Autodesk Inventor part; units mm, degrees
ref_plane "YZ Plane" through (0, 0, 0) normal (1, 0, 0) x (0, 1, 0)
ref_plane "XZ Plane" through (0, 0, 0) normal (0, 1, 0) x (-1, 0, 0)
ref_plane "XY Plane" through (0, 0, 0) normal (0, 0, 1) x (1, 0, 0)
sketch "Sketch1" plane through (0, 0, 0) normal (0, 0, 1) x (1, 0, 0)
  line L0 (-4.55, 7.5) -> (4.55, 7.5)
  line L1 (4.55, 7.5) -> (4.55, -7.5)
  line L2 (4.55, -7.5) -> (-4.55, -7.5)
  line L3 (-4.55, -7.5) -> (-4.55, 7.5)
  line L4 (-4.55, 7.5) -> (4.55, -7.5) construction
  line L5 (4.55, 7.5) -> (-4.55, -7.5) construction
  line L6 (-2.05, -2.05) -> (2.05, -2.05)
  line L7 (2.05, -2.05) -> (2.05, 2.05)
  line L8 (2.05, 2.05) -> (-2.05, 2.05)
  line L9 (-2.05, 2.05) -> (-2.05, -2.05)
  line L10 (-2.05, -2.05) -> (2.05, 2.05) construction
  line L11 (2.05, -2.05) -> (-2.05, 2.05) construction
  line L12 (-4.55, 7.5) -> (-16.55, 7.5)
  line L13 (-16.55, 7.5) -> (-16.55, 6)
  line L14 (-16.55, 6) -> (-4.55, 6)
  line L15 (-4.55, 6) -> (-4.55, 7.5)
  line L16 (-4.55, -7.5) -> (-16.55, -7.5)
  line L17 (-16.55, -7.5) -> (-16.55, -6)
  line L18 (-16.55, -6) -> (-4.55, -6)
  line L19 (-4.55, -6) -> (-4.55, -7.5)
  line L20 (4.55, 7.5) -> (16.55, 7.5)
  line L21 (16.55, 7.5) -> (16.55, 6)
  line L22 (16.55, 6) -> (4.55, 6)
  line L23 (4.55, 6) -> (4.55, 7.5)
  line L24 (4.55, -7.5) -> (16.55, -7.5)
  line L25 (16.55, -7.5) -> (16.55, -6)
  line L26 (16.55, -6) -> (4.55, -6)
  line L27 (4.55, -6) -> (4.55, -7.5)
  point P0 (0, 0)
  point P1 (-4.55, 6)
  point P2 (-4.55, -6)
  point P3 (4.55, 6)
  dimension "d0" = 15
  dimension "d1" = 9.1
  dimension "d2" = 4.1
  dimension "d3" = 4.1
  dimension "d4" = 12
  dimension "d5" = 1.5
  dimension "d8" = 1.5
  dimension "d9" = 12
  dimension "d10" = 12
  dimension "d11" = 1.5
  dimension "d12" = 12
extrude "Extrusion1" add sketch "Sketch1" along normal blind 10
sketch "Sketch2" plane through (0, 0, 10) normal (0, 0, 1) x (1, 0, 0)
  point P0 (0, 0)
fillet "Fillet1" radius 2 8 edges at (-16.55, 6.75, 10) (-16.55, -6.75, 10) (16.55, -6.75, 10) (16.55, 6.75, 10) (16.55, 6.75, 0) (-16.55, 6.75, 0) (-16.55, -6.75, 0) (16.55, -6.75, 0)
sketch "Sketch3" plane through (0, 0, 0) normal (0, 0, -1) x (-1, 0, 0)
  line L0 (-2.05, 5.05) -> (2.05, 5.05)
  line L1 (2.05, 5.05) -> (2.05, 3.55)
  line L2 (2.05, 3.55) -> (-2.05, 3.55)
  line L3 (-2.05, 3.55) -> (-2.05, 5.05)
  line L4 (-2.05, -3.55) -> (2.05, -3.55)
  line L5 (2.05, -3.55) -> (2.05, -5.05)
  line L6 (2.05, -5.05) -> (-2.05, -5.05)
  line L7 (-2.05, -5.05) -> (-2.05, -3.55)
  line L8 (-2.05, 2.05) -> (-2.05, -2.05)
  line L9 (2.05, -2.05) -> (2.05, 2.05)
  line L10 (2.05, 2.05) -> (-2.05, 2.05)
  line L11 (-2.05, -2.05) -> (2.05, -2.05)
  point P0 (0, 0)
  dimension "d16" = 1.5
  dimension "d17" = 1.5
  dimension "d18" = 1.5
  dimension "d19" = 1.5
extrude "Extrusion2" cut sketch "Sketch3" against normal blind 10 contours L0 L1 L2 L3 | L4 L5 L6 L7
properties part number "fuselage_tail_interface_back"
Verification items for the finished model (mm, model axes). A direction names the side the tool comes from. Give positions to 0.01 mm unless a question says otherwise; leave off trailing zeros. Order: outer loops, then holes, each group sorted by start corner. A loop starts at its lowest first (then second) coordinate and runs counter-clockwise, first axis right, second up. Notation, with made-up numbers: (6, 84) -> (48, 84) arc R17 ccw to (48, 105) -> close; hole circle Ø2 at (23.25, -24). An arc over 180 degrees is marked (long way). One line per item, written item: value.
(1) Sectioned sample at D-D on x = 13. Record the cut outline in (y, z), then the cut area to 3 significant figures.
Final values:
outline: (-7.5, 0) -> (-6, 0) -> (-6, 10) -> (-7.5, 10) -> close; (6, 0) -> (7.5, 0) -> (7.5, 10) -> (6, 10) -> close
area: 30.0 mm^2
(2) Tool access check on faces 1 (the face through (16.55, 7, 5)), 2 (the face through (-16.55, 7, 5)), 3 (the face through (-4.55, 0, 5)), 4 (the face through (0, -2.05, 5)), 5 (the face through (11, 6, 5)). Record the directions out of +Z, -Z, +X, -X, +Y, -Y that give a thin tool (end or side, any length) a straight path to the whole face; none if there is none.
Final values:
face 1: +Z, -Z, +X, +Y, -Y
face 2: +Z, -Z, -X, +Y, -Y
face 3: +Z, -Z, -X
face 4: +Z, -Z
face 5: +Z, -Z, +X
(3) Sectioned sample at B-B on x = 1. Record the cut outline in (y, z), then the cut area to 3 significant figures.
Final values:
outline: (-7.5, 0) -> (-5.05, 0) -> (-5.05, 10) -> (-7.5, 10) -> close; (-3.55, 0) -> (-2.05, 0) -> (-2.05, 10) -> (-3.55, 10) -> close; (2.05, 0) -> (3.55, 0) -> (3.55, 10) -> (2.05, 10) -> close; (5.05, 0) -> (7.5, 0) -> (7.5, 10) -> (5.05, 10) -> close
area: 79.0 mm^2
(4) Gauge pin test, flat ends, axial feed: pin 1 (0.8 mm diameter, centred on y = -4.5, z = 4, fed in from +X); pin 2 (3 mm diameter, centred on y = -0.5, z = 4, fed in from -X). Record the tip position at first contact, or that the pin passes through.
Final values:
pin 1: x = 4.55
pin 2: x = -4.55
(5) Sectioned sample at C-C on y = 4.25. Record the cut outline in (x, z).
Final values:
outline: (-4.55, 0) -> (-2.05, 0) -> (-2.05, 10) -> (-4.55, 10) -> close; (2.05, 0) -> (4.55, 0) -> (4.55, 10) -> (2.05, 10) -> close
(6) Scan lines: line 1 along Y through (x, z) = (-0.5, 6.75); line 2 along X through (y, z) = (0.25, 7.5); line 3 along Y through (x, z) = (13, 8.5). Record each from-to range of solid material in increasing order. Write a range as [from, to].
Final values:
line 1: [-7.5, -5.05], [-3.55, -2.05], [2.05, 3.55], [5.05, 7.5]
line 2: [-4.55, -2.05], [2.05, 4.55]
line 3: [-7.5, -6], [6, 7.5]
(7) Sectioned sample at A-A on z = 6.25. Record the cut outline in (x, y), then the cut area to 3 significant figures.
Final values:
outline: (-16.55, -7.5) -> (16.55, -7.5) -> (16.55, -6) -> (4.55, -6) -> (4.55, 6) -> (16.55, 6) -> (16.55, 7.5) -> (-16.55, 7.5) -> (-16.55, 6) -> (-4.55, 6) -> (-4.55, -6) -> (-16.55, -6) -> close; hole (-2.05, -5.05) -> (2.05, -5.05) -> (2.05, -3.55) -> (-2.05, -3.55) -> close; hole (-2.05, -2.05) -> (2.05, -2.05) -> (2.05, 2.05) -> (-2.05, 2.05) -> close; hole (-2.05, 3.55) -> (2.05, 3.55) -> (2.05, 5.05) -> (-2.05, 5.05) -> close
area: 179 mm^2
(8) Draft check along X on faces 6 (the face through (-2.05, -4, 5)), 7 (the face through (15.95, -6.74, 9.43)), 8 (the face through (0, 7.5, 5)). Enter one of: pulls with the +X half, pulls with the -X half, needs draft (parallel to the pull), parting line crosses it, or undercut.
Final values:
face 6: undercut
face 7: pulls with the +X half
face 8: needs draft
